The model under review builds one solid part; all positions refer to its coordinate system, in mm. A direction names the side the tool comes from. Coordinates: 2 decimals unless noted, no trailing zeros. Write each loop counter-clockwise with the first axis right and the second up, starting at its lowest first coordinate (ties: lowest second). Pieces come first, ordered by that corner, then holes. Notation, with made-up numbers: (-39, 63.5) - (-5, 63.5) arc R22 cw to (-5, 86.5) - close; hole circle Ø10 at (-10, -22). An arc over 180 degrees is marked (long way). Put each result on its own line as item: value. Start each with the question number.
Item 1: Mouldability with a two-part tool opening along X and no side actions: class faces 1 (the face through (7.034, 2.215, -0.986)), 2 (the face through (-5, 2.2, 0)), 3 (the face through (-5.3, 0.1, -1)) as pulls with the +X half, pulls with the -X half, needs draft (parallel to the pull), parting line crosses it, or undercut.
Item 2: Consider section A-A on x = 0. Give the boundary of the cut face in (y, z) (3 decimals), then the cut area to 3 significant figures.
Item 3: For pin 1 (0.8 mm diameter, centred on y = -5.5, z = -1.5, fed in from -X), flat-tipped, find the tip position at first contact; note if it passes through.
Item 4: Machinability: for faces 4 (the face through (-5, 2.2, -2)), 5 (the face through (0, -6.8, -1)), which of the approach directions +Z, -Z, +X, -X, +Y, -Y give a long, thin tool a straight path to every point of the face, cutting with its end or side? Answer none if there is none.
Item 5: Consider section C-C on z = -0.3. Give the boundary of the cut face in (x, y) (3 decimals).
Item 6: Consider section B-B on y = 0. Give the boundary of the cut face in (x, z) (3 decimals), then the cut area to 3 significant figures.
Item 7: To check wall thickness, follow L1, parallel to Y at x = -3, z = -0.65; L2, parallel to X at y = -0.5, z = -0.5; L3, parallel to Y at x = -4, z = -0.75. State the ranges of each line that lie inside material, in increasing order. Write a range as [from, to].
```python
from build123d import *

# Parameters (mm, degrees)
SKETCH3_R           = 7.375
BOSS_EXTRUDE1_DEPTH = 2


with BuildPart() as part:
    # Sketch3 → Boss-Extrude1 (new body)
    with BuildSketch(Plane.XY):
        Circle(SKETCH3_R)
        with BuildLine():
            Line((-2.75, 6.219123732), (-2.75, 4.530728418))
            ThreePointArc((-2.75, 4.530728418), (-5.3, 0), (-2.75, -4.530728418))
            Line((-2.75, -4.530728418), (-2.75, -6.219123732))
            ThreePointArc((-2.75, -6.219123732), (0, -6.8), (2.75, -6.219123732))
            Line((2.75, -6.219123732), (2.75, -4.530728418))
            ThreePointArc((2.75, -4.530728418), (5.3, 0), (2.75, 4.530728418))
            Line((2.75, 4.530728418), (2.75, 6.219123732))
            ThreePointArc((2.75, 6.219123732), (0, 6.8), (-2.75, 6.219123732))
        make_face(mode=Mode.SUBTRACT)
    extrude(amount=-BOSS_EXTRUDE1_DEPTH)


solid = part.part
```
Report:
1. face 1: parting line crosses it
1. face 2: needs draft
1. face 3: undercut
2. outline: (-7.375, -2) - (-6.8, -2) - (-6.8, 0) - (-7.375, 0) - close; (6.8, -2) - (7.375, -2) - (7.375, 0) - (6.8, 0) - close
2. area: 2.30 mm²
3. pin 1: x = -5.33
4. face 4: -Z, +X, -X, +Y, -Y
4. face 5: +Z, -Z
5. outline: circle Ø14.75 at (0, 0); hole (-2.75, -6.219) arc R6.8 ccw to (2.75, -6.219) - (2.75, -4.531) arc R5.3 ccw to (2.75, 4.531) - (2.75, 6.219) arc R6.8 ccw to (-2.75, 6.219) - (-2.75, 4.531) arc R5.3 ccw to (-2.75, -4.531) - close
6. outline: (-7.375, -2) - (-5.3, -2) - (-5.3, 0) - (-7.375, 0) - close; (5.3, -2) - (7.375, -2) - (7.375, 0) - (5.3, 0) - close
6. area: 8.30 mm²
7. L1: [-6.74, -4.37], [4.37, 6.74]
7. L2: [-7.36, -5.28], [5.28, 7.36]
7. L3: [-6.2, -3.48], [3.48, 6.2]
